from build123d import *

# Parameters (mm, degrees)
F1_DEPTH  = 11
F2_W      = 15
F2_H      = 5
F3_DEPTH  = 2
F4_W      = 9
F4_H      = 4.5
F5_DEPTH  = 2
F6_W      = 14
F6_H      = 4.5
F6_W_2    = 8
F7_DEPTH  = 2
F8_W      = 5.5
F8_H      = 9.5
F9_DEPTH  = 2
F10_DEPTH = 0.5


with BuildPart() as f1:
    # F0 (on Top) → F1 (new body)
    with BuildSketch(Plane.XY):
        with BuildLine():
            Line((14, 18), (-14, 18))
            ThreePointArc((-14, 18), (-16.828427, 16.828427), (-18, 14))
            Line((-18, 14), (-18, -14))
            ThreePointArc((-18, -14), (-16.828427, -16.828427), (-14, -18))
            Line((-14, -18), (14, -18))
            ThreePointArc((14, -18), (16.828427, -16.828427), (18, -14))
            Line((18, -14), (18, 14))
            ThreePointArc((18, 14), (16.828427, 16.828427), (14, 18))
        make_face()
    extrude(amount=F1_DEPTH)

    # F2 (on face) → F3 (cut)
    with BuildSketch(Plane.XZ.offset(18)):
        with Locations((4.5, 6.5)):
            Rectangle(F2_W, F2_H)
    extrude(amount=-F3_DEPTH, mode=Mode.SUBTRACT)

    # F4 (on face) → F5 (cut)
    with BuildSketch(Plane.YZ.offset(18)):
        with Locations((-5.5, 6.25)):
            Rectangle(F4_W, F4_H)
    extrude(amount=-F5_DEPTH, mode=Mode.SUBTRACT)

    # F6 (on face) → F7 (cut)
    with BuildSketch(Plane(origin=(0, 18, 0), x_dir=(-1, 0, 0), z_dir=(0, 1, 0))):
        with Locations((-5, 6.15)):
            Rectangle(F6_W, F6_H)
        with Locations((8, 6.15)):
            Rectangle(F6_W_2, F6_H)
    extrude(amount=-F7_DEPTH, mode=Mode.SUBTRACT)

    # F8 (on face) → F9 (cut)
    with BuildSketch(Plane.XY.offset(11)):
        with Locations((-1.75, 1.25)):
            Rectangle(F8_W, F8_H)
    extrude(amount=-F9_DEPTH, mode=Mode.SUBTRACT)

    # F8 (on face) → F10 (cut)
    with BuildSketch(Plane.XY.offset(11)):
        Polygon((13.195144, 11.430887), (8.865017, 8.930887), (13.195144, 6.430887), align=None)
    extrude(amount=-F10_DEPTH, mode=Mode.SUBTRACT)


solid = f1.part
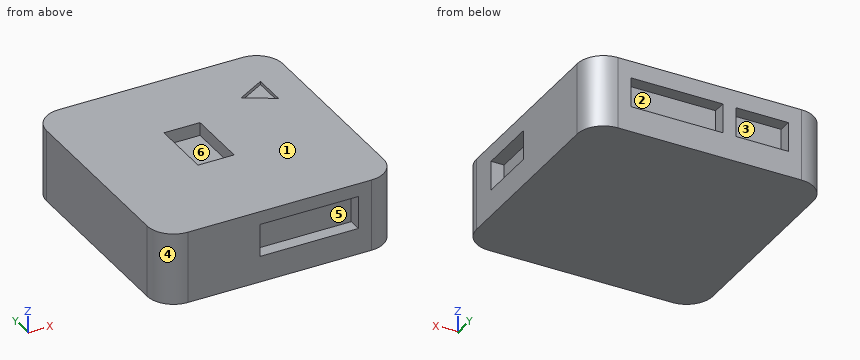
Geometry check sheet. Reference: the model listing, model coordinates, mm. Face numbers are marked on the shaded views. A direction names the side the tool comes from. Round coordinates to 2 decimals unless told otherwise and drop trailing zeros. Write each loop counter-clockwise with the first axis right and the second up, starting at its lowest first coordinate (ties: lowest second). Pieces come first, ordered by that corner, then holes. Notation, with made-up numbers: (-31, -37.75) -> (-22, -37.75) arc R20 cw to (-22, -20.75) -> close; hole circle Ø5 at (32, 70.25). An arc over 180 degrees is marked (long way). One line per item, written item: value. Start each with the question number.
(1) Access from +Z, -Z, +X, -X, +Y, -Y to the whole of each face (thin tool, end or side, straight path). Record for the marked faces 1 and 2.
(2) Scan lines: line 1 (Y direction, x = 5, z = 6); line 2 (X direction, y = -2.5, z = 6.25); line 3 (Z direction, x = 11, y = 9.5). Record each from-to range of solid material in increasing order. Write a range as [from, to].
(3) Draft check along Z on the marked faces 3, 4, 5 and 6. Enter one of: +Z half, -Z half, draft (parallel to the pull), parting line (faces both ways), or undercut.
(4) Cross-section at C-C, the plane z = 5.5. Record the cut outline in (x, y), and give its area (3 significant figures).
(5) Cross-section at B-B, the plane y = 2.5. Record the cut outline in (x, z).
(6) Cross-section at D-D, the plane x = -5. Record the cut outline in (y, z), and give its area (3 significant figures).
(7) Go/stop test with flat-tipped pins: pin 1 Ø1.6 at (y, z) = (17, 6.5) entering from -X; pin 2 Ø1.5 at (x, z) = (1, 7) entering from -Y; pin 3 Ø1.3 at (y, z) = (-5, 5.5) entering from +X. Record where each tip stops, or that it passes through.
(8) Cross-section at A-A, the plane z = 9.75. Record the cut outline in (x, y).
Answer:
1. face 1: +Z, +X, -X, +Y, -Y
1. face 2: +Y
2. line 1: [-16, 16]
2. line 2: [-18, 16]
2. line 3: [0, 10.5]
3. face 3: undercut
3. face 4: draft
3. face 5: undercut
3. face 6: +Z half
4. outline: (-18, -14) arc R4 ccw to (-14, -18) -> (-3, -18) -> (-3, -16) -> (12, -16) -> (12, -18) -> (14, -18) arc R4 ccw to (18, -14) -> (18, -10) -> (16, -10) -> (16, -1) -> (18, -1) -> (18, 14) arc R4 ccw to (14, 18) -> (12, 18) -> (12, 16) -> (-2, 16) -> (-2, 18) -> (-4, 18) -> (-4, 16) -> (-12, 16) -> (-12, 18) -> (-14, 18) arc R4 ccw to (-18, 14) -> close
4. area: 1,190 mm²
5. outline: (-18, 0) -> (18, 0) -> (18, 11) -> (1, 11) -> (1, 9) -> (-4.5, 9) -> (-4.5, 11) -> (-18, 11) -> close
6. outline: (-18, 0) -> (18, 0) -> (18, 3.9) -> (16, 3.9) -> (16, 8.4) -> (18, 8.4) -> (18, 11) -> (-18, 11) -> close
6. area: 387 mm²
7. pin 1: x = -17.34
7. pin 2: y = -16
7. pin 3: x = 16
8. outline: (-18, -14) arc R4 ccw to (-14, -18) -> (14, -18) arc R4 ccw to (18, -14) -> (18, 14) arc R4 ccw to (14, 18) -> (-14, 18) arc R4 ccw to (-18, 14) -> close; hole (-4.5, -3.5) -> (1, -3.5) -> (1, 6) -> (-4.5, 6) -> close
